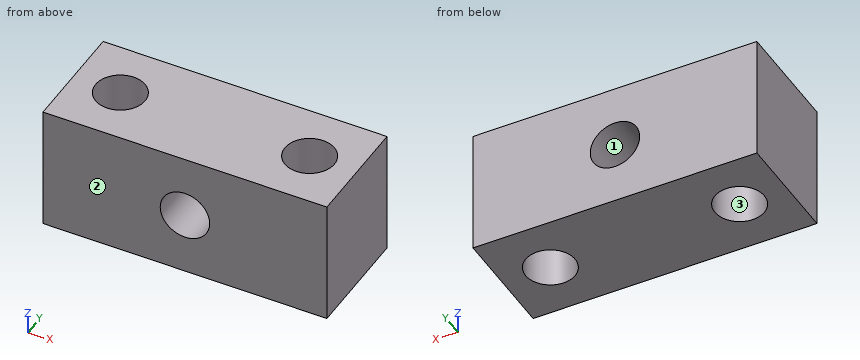
```python
from build123d import *

# Parameters (mm, degrees)
SKETCH1_R           = 2.4892
BOSS_EXTRUDE1_DEPTH = 6.35
SKETCH3_R           = 2.4892
CUT_EXTRUDE1_DEPTH  = 20.307713557


with BuildPart() as part:
    # Sketch1 → Boss-Extrude1 (new, symmetric)
    with BuildSketch(Plane.XY):
        Polygon((-9.525, -5.6642), (9.525, -5.6642), (14.2875, -5.6642), (14.2875, 5.6642), (9.525, 5.6642), (-9.525, 5.6642), (-14.2875, 5.6642), (-14.2875, -5.6642), align=None)
        with Locations((-9.525, 0)):
            Circle(SKETCH1_R, mode=Mode.SUBTRACT)
        with Locations((9.525, 0)):
            Circle(SKETCH1_R, mode=Mode.SUBTRACT)
    extrude(amount=BOSS_EXTRUDE1_DEPTH, both=True)

    # Sketch3 → Cut-Extrude1 (cut, through all)
    with BuildSketch(Plane(origin=(0, 5.6642, 0), x_dir=(1, 0, 0), z_dir=(0, 1, 0))):
        with Locations(Location((0, 0, 0), (0, 0, 180))):
            Circle(SKETCH3_R)
    extrude(amount=-CUT_EXTRUDE1_DEPTH, mode=Mode.SUBTRACT)


solid = part.part
```
The model under review builds one solid part; all positions refer to its coordinate system, in mm. Face numbers are marked on the shaded views. Coordinates: 2 decimals unless noted, no trailing zeros. Order: outer loops, then holes, each group sorted by start corner. A loop starts at its lowest first (then second) coordinate and runs counter-clockwise, first axis right, second up. Notation, with made-up numbers: (58, 10.25) -> (80, 10.25) arc R20 ccw to (80, 23.25) -> close; hole circle Ø4 at (29.25, 37). An arc over 180 degrees is marked (long way). Answer in a Markdown table with one row per item. Add a question column.
Item 1: We need section D-D on z = 4.75. Write out the cut boundary in (x, y) (1 decimal).
Item 2: We need section A-A on y = 0. Write out the cut boundary in (x, z).
Item 3: We need section B-B on x = 0. Write out the cut boundary in (y, z), plus the area to 3 significant figures.
Item 4: To check wall thickness, follow probe 1 along Z at (x, y) = (0, 2); probe 2 along X at (y, z) = (0.5, 4.5); probe 3 along X at (y, z) = (2.25, 2.25). State the ranges of each line that lie inside material, in increasing order.
Item 5: We need section C-C on z = 0. Write out the cut boundary in (x, y) (1 decimal), plus the area to 3 significant figures.
Item 6: Mouldability with a two-part tool opening along Y and no side actions: class the marked faces 1, 2 and 3 as +Y half, -Y half, draft (parallel to the pull), parting line (faces both ways), or undercut.
Final values:
| question | item | result |
|---|---|---|
| 1 | outline | (-14.3, -5.7) -> (14.3, -5.7) -> (14.3, 5.7) -> (-14.3, 5.7) -> close; hole circle Ø5 at (-9.5, 0); hole circle Ø5 at (9.5, 0) |
| 2 | outline | (-14.29, -6.35) -> (-12.01, -6.35) -> (-12.01, 6.35) -> (-14.29, 6.35) -> close; (-7.04, -6.35) -> (7.04, -6.35) -> (7.04, 6.35) -> (-7.04, 6.35) -> close; (12.01, -6.35) -> (14.29, -6.35) -> (14.29, 6.35) -> (12.01, 6.35) -> close; hole circle Ø4.98 at (0, 0) |
| 3 | outline | (-5.66, -6.35) -> (5.66, -6.35) -> (5.66, -2.49) -> (-5.66, -2.49) -> close; (-5.66, 2.49) -> (5.66, 2.49) -> (5.66, 6.35) -> (-5.66, 6.35) -> close |
| 3 | area | 87.5 mm2 |
| 4 | probe 1 | z = -6.35 to -2.49, 2.49 to 6.35 |
| 4 | probe 2 | x = -14.29 to -11.96, -7.09 to 7.09, 11.96 to 14.29 |
| 4 | probe 3 | x = -14.29 to -10.59, -8.46 to -1.06, 1.06 to 8.46, 10.59 to 14.29 |
| 5 | outline | (-14.3, -5.7) -> (-2.5, -5.7) -> (-2.5, 5.7) -> (-14.3, 5.7) -> close; (2.5, -5.7) -> (14.3, -5.7) -> (14.3, 5.7) -> (2.5, 5.7) -> close; hole circle Ø5 at (-9.5, 0); hole circle Ø5 at (9.5, 0) |
| 5 | area | 228 mm2 |
| 6 | face 1 | draft |
| 6 | face 2 | -Y half |
| 6 | face 3 | undercut |
